Verification items for the finished model (mm, model axes). A direction names the side the tool comes from. Coordinates: 2 decimals unless noted, no trailing zeros. Loops run counter-clockwise (first coordinate to the right, second up) from the corner with the lowest first, then second, coordinate; pieces in that order, holes last. Notation, with made-up numbers: (-26.5, 80) - (14.5, 80) arc R12 cw to (14.5, 84) - close; hole circle Ø8 at (74, -8.5). An arc over 180 degrees is marked (long way). Answer as CSV lines item,"result". Start each with the question number.
1. Cross-section at D-D (x = 2). Enter the section's corners in (y, z) (3 decimals).
2. Set-up check for faces 4 (the flat face through (-1, -8, 3.175)), 5 (the flat face through (6.35, 0, 2)): record each of +Z, -Z, +X, -X, +Y, -Y from which the full face is reachable in a straight line by a thin tool's end or side.
3. Cross-section at A-A (y = 0). Enter the section's corners in (x, z) (3 decimals).
4. Cross-section at C-C (x = -30.5). Enter the section's corners in (y, z) (3 decimals).
5. Material ranges on line 1 (Y direction, x = 0, z = 1.3) (3 decimals); line 2 (X direction, y = -4.5, z = 1.85); line 3 (X direction, y = 29, z = 1.25), recorded low to high. Write a range as [from, to].
6. Release check for a two-part mould opening along X. For faces 1 (the cylindrical face through (-5.291, 40.294, 1.565)), 2 (the flat face through (3.131, -5.525, 1.61)), 3 (the flat face through (-1, -8, 0)) record: pulls with the +X half, pulls with the -X half, needs draft (parallel to the pull), parting line crosses it, or undercut.
7. Cross-section at B-B (z = 1.2). Enter the section's corners in (x, y) (3 decimals), plus the area to 3 significant figures.
8. Gauge pin test, flat end, axial feed: P1, Ø11, axis at x = 32.893, y = 0, coming from the -Z side. Record the tip position at first contact, or that the pin passes through.
```python
from build123d import *

# Parameters (mm, degrees)
F0_R     = 40.64
F1_DEPTH = 3.175
F2_R     = 4.318
F4_DEPTH = 25.4
F5_DEPTH = 25.4


with BuildPart() as f1:
    # F0 (on Top) → F1 (new body)
    with BuildSketch(Plane.XY):
        Circle(F0_R)
    extrude(amount=F1_DEPTH)

    # F2 (on face) → F4 (cut)
    with BuildSketch(Plane.XY.offset(3.175)):
        with Locations((-32.893, 0)):
            Circle(F2_R)
        with Locations((0, -32.893)):
            Circle(F2_R)
        with Locations((32.893, 0)):
            Circle(F2_R)
        with Locations((0, 32.893)):
            Circle(F2_R)
    extrude(amount=-F4_DEPTH, mode=Mode.SUBTRACT)

    # F3 (on face) → F5 (cut)
    with BuildSketch(Plane.XY.offset(3.175)):
        Polygon((6.35, -3.666174), (6.35, 3.666174), (0, 7.332348), (-6.35, 3.666174), (-6.35, -3.666174), (0, -7.332348), align=None)
    extrude(amount=-F5_DEPTH, mode=Mode.SUBTRACT)


solid = f1.part
```
Values follow:
1,outline,"(-40.591, 0) - (-36.72, 0) - (-36.72, 3.175) - (-40.591, 3.175) - close; (-29.066, 0) - (-6.178, 0) - (-6.178, 3.175) - (-29.066, 3.175) - close; (6.178, 0) - (29.066, 0) - (29.066, 3.175) - (6.178, 3.175) - close; (36.72, 0) - (40.591, 0) - (40.591, 3.175) - (36.72, 3.175) - close"
2,face 4,"+Z, +X, -X, +Y, -Y"
2,face 5,"+Z, -Z"
3,outline,"(-40.64, 0) - (-37.211, 0) - (-37.211, 3.175) - (-40.64, 3.175) - close; (-28.575, 0) - (-6.35, 0) - (-6.35, 3.175) - (-28.575, 3.175) - close; (6.35, 0) - (28.575, 0) - (28.575, 3.175) - (6.35, 3.175) - close; (37.211, 0) - (40.64, 0) - (40.64, 3.175) - (37.211, 3.175) - close"
4,outline,"(-26.858, 0) - (-3.594, 0) - (-3.594, 3.175) - (-26.858, 3.175) - close; (3.594, 0) - (26.858, 0) - (26.858, 3.175) - (3.594, 3.175) - close"
5,line 1,"y = [-40.64, -37.211], [-28.575, -7.332], [7.332, 28.575], [37.211, 40.64]"
5,line 2,"x = [-40.39, -4.91], [4.91, 40.39]"
5,line 3,"x = [-28.47, -1.87], [1.87, 28.47]"
6,face 1,"parting line crosses it"
6,face 2,"undercut"
6,face 3,"needs draft"
7,outline,"circle Ø81.28 at (0, 0); hole circle Ø8.636 at (-32.893, 0); hole (-6.35, -3.666) - (0, -7.332) - (6.35, -3.666) - (6.35, 3.666) - (0, 7.332) - (-6.35, 3.666) - close; hole circle Ø8.636 at (0, -32.893); hole circle Ø8.636 at (0, 32.893); hole circle Ø8.636 at (32.893, 0)"
7,area,"4,810 mm²"
8,P1,"stops at z = 0"
